from build123d import *

# Parameters (mm, degrees)
F1_DEPTH  = 40
F2_T      = -2.5
F3_R      = 30.5
F4_DEPTH  = 5
F6_DEPTH  = 3
F7_W      = 40
F7_H      = 5
F8_DEPTH  = 5
F9_W      = 16
F9_H      = 5
F10_DEPTH = 5
F11_W     = 8
F11_H     = 4
F12_DEPTH = 2.5


with BuildPart() as f1:
    # F0 (on Front) → F1 (new body)
    with BuildSketch(Plane.XZ):
        with BuildLine():
            ThreePointArc((85, 30), (82.0710678119, 37.0710678119), (75, 40))
            Line((75, 40), (-75, 40))
            ThreePointArc((-75, 40), (-82.0710678119, 37.0710678119), (-85, 30))
            Line((-85, 30), (-85, -30))
            ThreePointArc((-85, -30), (-82.0710678119, -37.0710678119), (-75, -40))
            Line((-75, -40), (75, -40))
            ThreePointArc((75, -40), (82.0710678119, -37.0710678119), (85, -30))
            Line((85, -30), (85, 30))
        make_face()
    extrude(amount=F1_DEPTH)

    # F2
    f2_openings = [f1.faces().sort_by_distance(p)[0] for p in [
        (0, 0, 0),
    ]]
    offset(amount=F2_T, openings=f2_openings)

    # F3 (on face) → F4 (cut)
    with BuildSketch(Plane.XZ.offset(40)):
        with Locations((-50, 0)):
            Circle(F3_R)
        with Locations((50, 0)):
            Circle(F3_R)
    extrude(amount=-F4_DEPTH, mode=Mode.SUBTRACT)

    # F5 (on face) → F6 (join)
    with BuildSketch(Plane(origin=(0, 0, 0), x_dir=(-1, 0, 0), z_dir=(0, 1, 0))):
        with BuildLine():
            Line((-85, 30), (-85, -30))
            ThreePointArc((-85, -30), (-82.0710678119, -37.0710678119), (-75, -40))
            Line((-75, -40), (75, -40))
            ThreePointArc((75, -40), (82.0710678119, -37.0710678119), (85, -30))
            Line((85, -30), (85, 30))
            ThreePointArc((85, 30), (82.0710678119, 37.0710678119), (75, 40))
            Line((75, 40), (-75, 40))
            ThreePointArc((-75, 40), (-82.0710678119, 37.0710678119), (-85, 30))
        make_face()
        with BuildLine():
            Line((75, -37.5), (-75, -37.5))
            ThreePointArc((-75, -37.5), (-80.3033008589, -35.3033008589), (-82.5, -30))
            Line((-82.5, -30), (-82.5, 30))
            ThreePointArc((-82.5, 30), (-80.3033008589, 35.3033008589), (-75, 37.5))
            Line((-75, 37.5), (75, 37.5))
            ThreePointArc((75, 37.5), (80.3033008589, 35.3033008589), (82.5, 30))
            Line((82.5, 30), (82.5, -30))
            ThreePointArc((82.5, -30), (80.3033008589, -35.3033008589), (75, -37.5))
        make_face(mode=Mode.SUBTRACT)
        with BuildLine():
            ThreePointArc((-82.5, -30), (-80.3033008589, -35.3033008589), (-75, -37.5))
            Line((-75, -37.5), (75, -37.5))
            ThreePointArc((75, -37.5), (80.3033008589, -35.3033008589), (82.5, -30))
            Line((82.5, -30), (82.5, 30))
            ThreePointArc((82.5, 30), (80.3033008589, 35.3033008589), (75, 37.5))
            Line((75, 37.5), (-75, 37.5))
            ThreePointArc((-75, 37.5), (-80.3033008589, 35.3033008589), (-82.5, 30))
            Line((-82.5, 30), (-82.5, -30))
        make_face()
    extrude(amount=F6_DEPTH)

    # F7 (on face) → F8 (cut)
    with BuildSketch(Plane.XZ.offset(40)):
        with Locations((0, 18)):
            Rectangle(F7_W, F7_H)
    extrude(amount=-F8_DEPTH, mode=Mode.SUBTRACT)

    # F9 (on face) → F10 (cut)
    with BuildSketch(Plane.XZ.offset(40)):
        with Locations((0, -22)):
            Rectangle(F9_W, F9_H)
    extrude(amount=-F10_DEPTH, mode=Mode.SUBTRACT)

    # F11 (on face) → F12 (cut)
    with BuildSketch(Plane.XY.offset(40)):
        with Locations((0, -3)):
            Rectangle(F11_W, F11_H)
    extrude(amount=-F12_DEPTH, mode=Mode.SUBTRACT)


solid = f1.part
Build history of the part. All positions in model axes, mm. A direction names the side the tool comes from. Coordinates: 2 decimals unless noted, no trailing zeros. Order: outer loops, then holes, each group sorted by start corner. A loop starts at its lowest first (then second) coordinate and runs counter-clockwise, first axis right, second up. Notation, with made-up numbers: (85.25, 54) - (109.25, 54) arc R22 cw to (109.25, 76) - close; hole circle Ø4 at (-20.5, -6.75). An arc over 180 degrees is marked (long way). Write each question's results on one line, items separated by ' | '. Start each with the question number.
Item 1: Tool access for faces 4 (the face through (-82.5, -18, 0)), 5 (the face through (-21.826, -38.768, -11.682)), 6 (the face through (1, -19, -40)): list every direction of +Z, -Z, +X, -X, +Y, -Y with a clear straight run to the whole face (end or side of a thin tool).
Item 2: Wall check: probe 1 along Y at (x, z) = (-14, -17); probe 2 along Z at (x, y) = (27.5, -10); probe 3 along Z at (x, y) = (-50, -39). Give the ranges that are in metal, low to high. Write a range as [from, to].
Item 3: Band-saw the part on A-A on y = -11.5. Write the cut outline in (x, z), and give its area (3 significant figures).
Item 4: Band-saw the part on D-D on z = 33. Write the cut outline in (x, y), and give its area (3 significant figures).
Item 5: Band-saw the part on B-B on z = 0. Write the cut outline in (x, y).
Item 6: Mould opens along Z. For faces 1 (the face through (82.15, -18.8, -36.99)), 2 (the face through (-1, -18, -37.5)), 3 (the face through (1, 3, 1)) say: released by +Z, released by -Z, zero draft, split by the parting line, or undercut.
Item 7: Flat gauge pins, fed straight in: pin 1 (2 mm diameter, centred on y = -2.5, z = 39, fed in from -X); pin 2 (12 mm diameter, centred on x = -53.5, z = -10.5, fed in from -Y); pin 3 (3 mm diameter, centred on y = -2.5, z = 38.5, fed in from +X). Where does each tip first touch, or does it go through?
Item 8: Band-saw the part on C-C on x = -50. Write the cut outline in (y, z), and give its area (3 significant figures).
Numbers:
1) face 4: none | face 5: -Y | face 6: -Z, +X, -X, +Y, -Y
2) probe 1: [-40, -37.5], [0, 3] | probe 2: [-40, -37.5], [37.5, 40] | probe 3: [-40, -30.5], [30.5, 40]
3) outline: (-85, -30) arc R10 ccw to (-75, -40) - (75, -40) arc R10 ccw to (85, -30) - (85, 30) arc R10 ccw to (75, 40) - (-75, 40) arc R10 ccw to (-85, 30) - close; hole (-82.5, -30) arc R7.5 ccw to (-75, -37.5) - (75, -37.5) arc R7.5 ccw to (82.5, -30) - (82.5, 30) arc R7.5 ccw to (75, 37.5) - (-75, 37.5) arc R7.5 ccw to (-82.5, 30) - close | area: 1,190 mm^2
4) outline: (-84.54, -40) - (84.54, -40) - (84.54, 3) - (-84.54, 3) - close; hole (-81.87, -37.5) - (81.87, -37.5) - (81.87, 0) - (-81.87, 0) - close | area: 1,130 mm^2
5) outline: (-85, -40) - (-80.5, -40) - (-80.5, -37.5) - (-82.5, -37.5) - (-82.5, 0) - (82.5, 0) - (82.5, -37.5) - (80.5, -37.5) - (80.5, -40) - (85, -40) - (85, 3) - (-85, 3) - close; (-19.5, -40) - (19.5, -40) - (19.5, -37.5) - (-19.5, -37.5) - close
6) face 1: released by -Z | face 2: undercut | face 3: zero draft
7) pin 1: x = -81 | pin 2: y = 0 | pin 3: x = 82.14
8) outline: (-40, -40) - (3, -40) - (3, 40) - (-40, 40) - (-40, 30.5) - (-37.5, 30.5) - (-37.5, 37.5) - (0, 37.5) - (0, -37.5) - (-37.5, -37.5) - (-37.5, -30.5) - (-40, -30.5) - close | area: 475 mm^2
